```python
from build123d import *

# Parameters (mm, degrees)
SKETCH_2_R          = 19
SKETCH_2_R_2        = 2.75
EXTRUDE_1_DEPTH     = 13.9
SKETCH_3_R          = 21.125
CUT_EXTRUDE_1_DEPTH = 12.15
SKETCH_4_R          = 5
CUT_EXTRUDE_2_DEPTH = 3
FILLET_1_R          = 8
SKETCH_5_R          = 0.9
CUT_EXTRUDE_3_DEPTH = 60.993937194


with BuildPart() as part:
    # Эскиз2 → Бобышка-Вытянуть1 (new body)
    with BuildSketch(Plane.XY):
        with BuildLine():
            ThreePointArc((26, 26.25), (0, 52.25), (-26, 26.25))
            Line((-26, 26.25), (-26, -20))
            Line((-26, -20), (26, -20))
            Line((26, -20), (26, 26.25))
        make_face()
        with Locations((0, 26.25)):
            Circle(SKETCH_2_R, mode=Mode.SUBTRACT)
        with Locations((12, -10)):
            Circle(SKETCH_2_R_2, mode=Mode.SUBTRACT)
        with Locations((-12, -10)):
            Circle(SKETCH_2_R_2, mode=Mode.SUBTRACT)
    extrude(amount=EXTRUDE_1_DEPTH)

    # Эскиз3 → Вырез-Вытянуть1 (cut)
    with BuildSketch(Plane.XY.offset(13.9)):
        with Locations((0, 26.25)):
            Circle(SKETCH_3_R)
    extrude(amount=-CUT_EXTRUDE_1_DEPTH, mode=Mode.SUBTRACT)

    # Эскиз4 → Вырез-Вытянуть2 (cut)
    with BuildSketch(Plane(origin=(0, 0, 0), x_dir=(-1, 0, 0), z_dir=(0, 0, -1))):
        with Locations((-12, -10)):
            Circle(SKETCH_4_R)
        with Locations((12, -10)):
            Circle(SKETCH_4_R)
    extrude(amount=-CUT_EXTRUDE_2_DEPTH, mode=Mode.SUBTRACT)

    # Скругление1
    fillet_1_edges = [part.edges().sort_by_distance(p)[0] for p in [
        (26, -20, 6.95),
        (-26, -20, 6.95),
    ]]
    fillet(fillet_1_edges, radius=FILLET_1_R)

    # Эскиз5 → Вырез-Вытянуть3 (cut, through all)
    with BuildSketch(Plane.XY.offset(13.9)):
        with Locations((0, 49.75)):
            Circle(SKETCH_5_R)
        with Locations((-23.5, 26.25)):
            Circle(SKETCH_5_R)
        with Locations((0, 2.75)):
            Circle(SKETCH_5_R)
        with Locations((23.5, 26.25)):
            Circle(SKETCH_5_R)
        with Locations((-22, -10)):
            Circle(SKETCH_5_R)
        with Locations(Location((22, -10, 0), (0, 0, 180))):
            Circle(SKETCH_5_R)
    extrude(amount=-CUT_EXTRUDE_3_DEPTH, mode=Mode.SUBTRACT)


solid = part.part
```
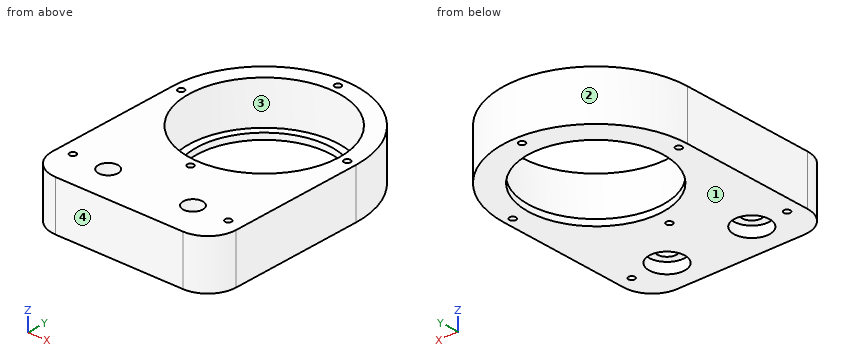
Here's how the part is built. I have some questions about the finished solid (model axes, mm). Face numbers are marked on the shaded views. Round coordinates to 2 decimals unless told otherwise and drop trailing zeros. Order: outer loops, then holes, each group sorted by start corner. A loop starts at its lowest first (then second) coordinate and runs counter-clockwise, first axis right, second up. Notation, with made-up numbers: (-14, 31.5) -> (27, 31.5) arc R18 ccw to (27, 53.5) -> close; hole circle Ø7 at (-11.5, 15). An arc over 180 degrees is marked (long way). Use a Markdown table: item, result. Add a question column.
(1) Suppose I cut it at A-A, the plane y = -10. Please give me the cut outline in (x, z).
(2) If we mould it in two halves opening along Y, with no side actions, what happens to the marked faces 1, 2, 3 and 4? For each: released by +Y, released by -Y, zero draft, split by the parting line, or undercut.
(3) For pin 1 Ø1.6 at (x, y) = (-23.5, 26.25) entering from +Z; pin 2 Ø5 at (y, z) = (40.5, 3.5) entering from -X; pin 3 Ø3 at (x, y) = (-14.5, 37) entering from +Z; pin 4 Ø4 at (y, z) = (30, 12) entering from -X, each with a flat end and sliding along its axis, tell me the tip position at first contact or that it passes through.
(4) Suppose I cut it at B-B, the plane z = 5. Count the separate pieces of the cut face and the enclosed holes in it, and give its area (3 significant figures).
(5) I need wall thicknesses on line 1 along Y through (x, z) = (0, 0.95); line 2 along Y through (x, z) = (0, 4.5) (3 decimals); line 3 along Y through (x, z) = (10, 5.75). Which ranges of each line are inside material? Lowest first, please.
(6) Suppose I cut it at C-C, the plane x = 0. Please give me the cut outline in (y, z) (3 decimals).
(7) Suppose I cut it at D-D, the plane x = 12. Please give me the cut outline in (y, z).
Verdict:
| question | item | result |
|---|---|---|
| 1 | outline | (-26, 0) -> (-22.9, 0) -> (-22.9, 13.9) -> (-26, 13.9) -> close; (-21.1, 0) -> (-17, 0) -> (-17, 3) -> (-14.75, 3) -> (-14.75, 13.9) -> (-21.1, 13.9) -> close; (-9.25, 3) -> (-7, 3) -> (-7, 0) -> (7, 0) -> (7, 3) -> (9.25, 3) -> (9.25, 13.9) -> (-9.25, 13.9) -> close; (14.75, 3) -> (17, 3) -> (17, 0) -> (21.1, 0) -> (21.1, 13.9) -> (14.75, 13.9) -> close; (22.9, 0) -> (26, 0) -> (26, 13.9) -> (22.9, 13.9) -> close |
| 2 | face 1 | zero draft |
| 2 | face 2 | released by +Y |
| 2 | face 3 | undercut |
| 2 | face 4 | released by -Y |
| 3 | pin 1 | through |
| 3 | pin 2 | x = -23.19 |
| 3 | pin 3 | z = 1.75 |
| 3 | pin 4 | x = -25.94 |
| 4 | separate pieces | 1 |
| 4 | enclosed holes | 9 |
| 4 | area | 1,970 mm2 |
| 5 | line 1 | -20 to 1.85, 3.65 to 7.25, 45.25 to 48.85, 50.65 to 52.25 |
| 5 | line 2 | -20 to 1.85, 3.65 to 5.125, 47.375 to 48.85, 50.65 to 52.25 |
| 5 | line 3 | -20 to -11.89, -8.11 to 7.64, 44.86 to 50.25 |
| 6 | outline | (-20, 0) -> (1.85, 0) -> (1.85, 13.9) -> (-20, 13.9) -> close; (3.65, 0) -> (7.25, 0) -> (7.25, 1.75) -> (5.125, 1.75) -> (5.125, 13.9) -> (3.65, 13.9) -> close; (45.25, 0) -> (48.85, 0) -> (48.85, 13.9) -> (47.375, 13.9) -> (47.375, 1.75) -> (45.25, 1.75) -> close; (50.65, 0) -> (52.25, 0) -> (52.25, 13.9) -> (50.65, 13.9) -> close |
| 7 | outline | (-20, 0) -> (-15, 0) -> (-15, 3) -> (-12.75, 3) -> (-12.75, 13.9) -> (-20, 13.9) -> close; (-7.25, 3) -> (-5, 3) -> (-5, 0) -> (11.52, 0) -> (11.52, 1.75) -> (8.86, 1.75) -> (8.86, 13.9) -> (-7.25, 13.9) -> close; (40.98, 0) -> (49.32, 0) -> (49.32, 13.9) -> (43.64, 13.9) -> (43.64, 1.75) -> (40.98, 1.75) -> close |
